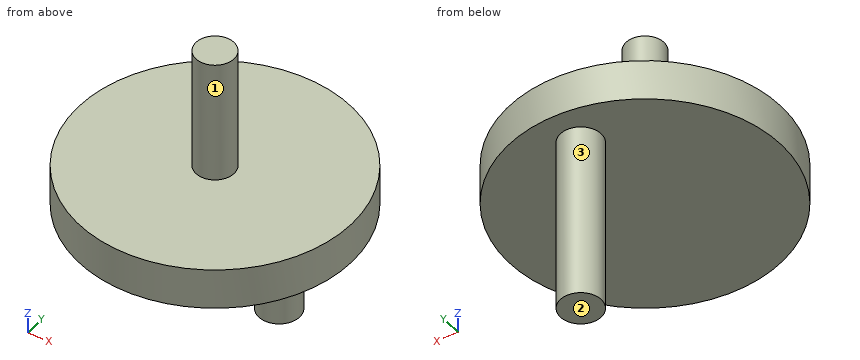
```python
from build123d import *

# Parameters (mm, degrees)
SKETCH1_R           = 50
SKETCH1_R_2         = 7.5
BOSS_EXTRUDE1_DEPTH = 15
SKETCH2_R           = 7.5
BOSS_EXTRUDE2_DEPTH = 80
SKETCH5_R           = 7
BOSS_EXTRUDE3_DEPTH = 45


with BuildPart() as part:
    # Sketch1 → Boss-Extrude1 (new body)
    with BuildSketch(Plane.XY):
        Circle(SKETCH1_R)
        with Locations((0, 35)):
            Circle(SKETCH1_R_2, mode=Mode.SUBTRACT)
    extrude(amount=BOSS_EXTRUDE1_DEPTH)

    # Sketch2 → Boss-Extrude2 (add)
    with BuildSketch(Plane.XY.offset(15)):
        with Locations((0, 35)):
            Circle(SKETCH2_R)
    extrude(amount=-BOSS_EXTRUDE2_DEPTH)

    # Sketch5 → Boss-Extrude3 (add)
    with BuildSketch(Plane.XY.offset(15)):
        Circle(SKETCH5_R)
    extrude(amount=BOSS_EXTRUDE3_DEPTH)


solid = part.part
```
Model file for the job. Use its own axes, mm. Face numbers are marked on the shaded views. A direction names the side the tool comes from. Give positions to 0.01 mm unless a question says otherwise; leave off trailing zeros. Order: outer loops, then holes, each group sorted by start corner. A loop starts at its lowest first (then second) coordinate and runs counter-clockwise, first axis right, second up.
1) Saw through at C-C, the plane z = 12.5. Write the cut outline in (x, y), then the cut area to 3 significant figures.
2) Wall check: probe 1 along Z at (x, y) = (-38.5, 16.5); probe 2 along Z at (x, y) = (-5, 30.5); probe 3 along X at (y, z) = (1, 18.5). Give the ranges that are in metal, low to high.
3) 3-axis set-ups, long thin cutter, end or side, ignore diameter. For the marked faces 1, 2 and 3: which of +Z, -Z, +X, -X, +Y, -Y reach the whole face in a straight line?
4) Saw through at D-D, the plane y = 35. Write the cut outline in (x, z), then the cut area to 3 significant figures.
5) Saw through at B-B, the plane y = 0. Write the cut outline in (x, z).
6) Pin check, flat tips, straight feed: pin 1 (8 mm diameter, centred on y = -10, z = 2, fed in from -X); pin 2 (4 mm diameter, centred on x = 1.5, z = -20.5, fed in from -Y); pin 3 (5 mm diameter, centred on y = 8, z = 34.5, fed in from -X). Stop position of each tip, or through.
7) Saw through at A-A, the plane x = 0. Write the cut outline in (y, z), then the cut area to 4 significant figures.
Computed:
1. outline: circle Ø100 at (0, 0)
1. area: 7,850 mm2
2. probe 1: z = 0 to 15
2. probe 2: z = -65 to 15
2. probe 3: x = -6.93 to 6.93
3. face 1: +Z
3. face 2: -Z, +X, -X, +Y, -Y
3. face 3: -Z
4. outline: (-35.71, 0) - (-7.5, 0) - (-7.5, -65) - (7.5, -65) - (7.5, 0) - (35.71, 0) - (35.71, 15) - (-35.71, 15) - close
4. area: 2,050 mm2
5. outline: (-50, 0) - (50, 0) - (50, 15) - (7, 15) - (7, 60) - (-7, 60) - (-7, 15) - (-50, 15) - close
6. pin 1: stops at x = -49.64
6. pin 2: stops at y = 27.5
6. pin 3: stops at x = -4.33
7. outline: (-50, 0) - (27.5, 0) - (27.5, -65) - (42.5, -65) - (42.5, 0) - (50, 0) - (50, 15) - (7, 15) - (7, 60) - (-7, 60) - (-7, 15) - (-50, 15) - close
7. area: 3,105 mm2
